Can you work these out from the model? Positions are in its coordinate system, mm. Coordinates: 2 decimals unless noted, no trailing zeros. Loops run counter-clockwise (first coordinate to the right, second up) from the corner with the lowest first, then second, coordinate; pieces in that order, holes last. Notation, with made-up numbers: (58.25, 44) -> (95.25, 44) arc R22 ccw to (95.25, 64) -> close; hole circle Ø1 at (-9, 72.25). An arc over 180 degrees is marked (long way). Put each result on its own line as item: value. Start each with the question number.
Item 1: Will this pin go through, and if not, where does the flat tip stop? P1, Ø3, axis at y = 1.5, z = 1, coming from the +X side.
Item 2: We'd pull the mould along X, two halves only. Please class faces 1 (the cylindrical face through (-1.43, -0.45, 0.04)), 2 (the cylindrical face through (0.434, 1.952, 2.494)): pulls with the +X half, pulls with the -X half, needs draft (parallel to the pull), parting line crosses it, or undercut.
Item 3: If we section it at C-C on z = 2.45: Please give me the cut outline in (x, y).
Item 4: Please list where these lines run through material, in increasing order: L1, parallel to X at y = -1.2, z = -0.05; L2, parallel to X at y = 0.25, z = -0.15; L3, parallel to Y at x = 0.55, z = -1.5. Write a range as from..to.
Item 5: If we section it at D-D on y = -1.9: Please give me the cut outline in (x, z).
Item 6: If we section it at A-A on y = 0: Please give me the cut outline in (x, z).
```python
from build123d import *


with BuildPart() as part:
    # Эскиз1 → Повернуть1 (revolve)
    with BuildSketch(Plane(origin=(0, 0, 0), x_dir=(1, 0, 0), z_dir=(0, 1, 0)), mode=Mode.PRIVATE) as revolve_1_sk:
        with BuildLine():
            Line((2, 2.9), (1.5, 2.9))
            Line((1.5, 2.9), (1.5, 2.481934729))
            ThreePointArc((1.5, 2.481934729), (1.760388745, 2.304567522), (2, 2.1))
            Line((2, 2.1), (2, 2.9))
        make_face()
        with BuildLine():
            ThreePointArc((2, 2.1), (1.760388745, 2.304567522), (1.5, 2.481934729))
            Line((1.5, 2.481934729), (1.5, -2.481934729))
            ThreePointArc((1.5, -2.481934729), (1.760388745, -2.304567522), (2, -2.1))
            Line((2, -2.1), (2, 2.1))
        make_face()
        with BuildLine():
            ThreePointArc((2, -2.1), (1.760388745, -2.304567522), (1.5, -2.481934729))
            Line((1.5, -2.481934729), (1.5, -2.9))
            Line((1.5, -2.9), (2, -2.9))
            Line((2, -2.9), (2, -2.1))
        make_face()
        with BuildLine():
            ThreePointArc((2.9, 0), (2.665520587, 1.142365966), (2, 2.1))
            Line((2, 2.1), (2, -2.1))
            ThreePointArc((2, -2.1), (2.665520587, -1.142365966), (2.9, 0))
        make_face()
    revolve(revolve_1_sk.sketch.rotate(Axis((0, 0, -3.556975885), (0, 0, 1)), 180), axis=Axis((0, 0, -3.556975885), (0, 0, 1)))


solid = part.part
```
Solutions:
1. P1: x = 2.88
2. face 1: undercut
2. face 2: parting line crosses it
3. outline: circle Ø4 at (0, 0); hole circle Ø3 at (0, 0)
4. L1: -2.64..-0.9, 0.9..2.64
4. L2: -2.89..-1.48, 1.48..2.89
4. L3: -2.42..-1.4, 1.4..2.42
5. outline: (-0.62, -2.9) -> (0.62, -2.9) -> (0.62, -2.1) arc R2.19 ccw to (0.62, 2.1) -> (0.62, 2.9) -> (-0.62, 2.9) -> (-0.62, 2.1) arc R2.19 ccw to (-0.62, -2.1) -> close
6. outline: (-2, -2.9) -> (-1.5, -2.9) -> (-1.5, 2.9) -> (-2, 2.9) -> (-2, 2.1) arc R2.9 ccw to (-2, -2.1) -> close; (1.5, -2.9) -> (2, -2.9) -> (2, -2.1) arc R2.9 ccw to (2, 2.1) -> (2, 2.9) -> (1.5, 2.9) -> close
